Source: CAD feature listing. Evaluate the final solid. Frame: model axes, mm. A direction names the side the tool comes from. Round coordinates to 2 decimals unless told otherwise and drop trailing zeros. Loops run counter-clockwise (first coordinate to the right, second up) from the corner with the lowest first, then second, coordinate; pieces in that order, holes last. Notation, with made-up numbers: M 89,-39.75 L 136,-39.75 A12 cw 136,-30.75 Z; hole C 84,71 d4. An arc over 180 degrees is marked long. Answer as a JSON object with one key per item and string values.
from build123d import *

# Parameters (mm, degrees)
F1_DEPTH  = 15
F0_W      = 5
F0_H      = 13.750002
F2_DEPTH  = 12.5
F4_R      = 5
F5_R      = 5
F6_R      = 5
F7_R      = 3.275
F8_DEPTH  = 25
F3_W      = 2.5
F3_H      = 2
F9_DEPTH  = 50
F10_R     = 5
F11_DEPTH = 30


with BuildPart() as f1:
    # F0 (on Front) → F1 (new body, symmetric)
    with BuildSketch(Plane.XZ):
        Polygon((6.421984, -16.497303), (-11.078016, -16.497303), (-10.973849, -22.747303), (29.026151, -22.747303), (29.026151, -16.497303), (11.421984, -16.497303), align=None)
    extrude(amount=F1_DEPTH, both=True)

    # F0 (on Front) → F2 (join, symmetric)
    with BuildSketch(Plane.XZ):
        Polygon((6.421984, -16.497303), (-11.078016, -16.497303), (-10.973849, -22.747303), (29.026151, -22.747303), (29.026151, -16.497303), (11.421984, -16.497303), align=None)
        with Locations((8.921984, -9.622302)):
            Rectangle(F0_W, F0_H)
    extrude(amount=F2_DEPTH, both=True)

    # F4
    f4_edges = [f1.edges().sort_by_distance(p)[0] for p in [
        (29.026151, -15, -19.622303),
    ]]
    fillet(f4_edges, radius=F4_R)

    # F5
    f5_edges = [f1.edges().sort_by_distance(p)[0] for p in [
        (29.026151, 15, -19.622303),
        (-11.025932, -15, -19.622303),
        (-11.025932, 15, -19.622303),
    ]]
    fillet(f5_edges, radius=F5_R)

    # F6
    f6_edges = [f1.edges().sort_by_distance(p)[0] for p in [
        (8.921984, 12.5, -2.747301),
        (8.921984, -12.5, -2.747301),
    ]]
    fillet(f6_edges, radius=F6_R)

    # F7 (on Top) → F8 (cut)
    with BuildSketch(Plane.XY):
        with Locations((22.092594, 8.45)):
            Circle(F7_R)
        with Locations((21.753448, -8.45)):
            Circle(F7_R)
    extrude(amount=-F8_DEPTH, mode=Mode.SUBTRACT)

    # F3 (on Front) → F9 (cut, symmetric)
    with BuildSketch(Plane.XZ):
        with Locations((-0.973849, -21.747303)):
            Rectangle(F3_W, F3_H)
    extrude(amount=F9_DEPTH, both=True, mode=Mode.SUBTRACT)

    # F10 (on Right) → F11 (cut, symmetric)
    with BuildSketch(Plane.YZ):
        with Locations((0, -9.563591)):
            Circle(F10_R)
    extrude(amount=F11_DEPTH, both=True, mode=Mode.SUBTRACT)


solid = f1.part
Item 1: Contact query for flat-ended pins moving along their axis: pin 1 Ø11 at (y, z) = (-4, -10) entering from -X; pin 2 Ø8.5 at (x, y) = (21.75, -8.45) entering from +Z; pin 3 Ø0.6 at (y, z) = (7, -21.5) entering from -X; pin 4 Ø9 at (y, z) = (0, -9.56) entering from -X. Output: stop coordinate, or through.
Answer sheet:
{"pin 1": "stops at x = 6.42", "pin 2": "stops at z = -16.5", "pin 3": "stops at x = -11", "pin 4": "passes through"}
Item 2: Section D-D on x = -5.5. Return the cut outline in (y, z), then the cut area to 4 significant figures.
Answer sheet:
{"outline": "M -15,-22.75 L 15,-22.75 L 15,-16.5 L -15,-16.5 Z", "area": "187.5 mm²"}
Item 3: Pull-direction query (Y, two-part tool) for faces 4 (the cylindrical face through (8.957, -1.084, -14.445)), 5 (the cylindrical face through (-9.521, 13.574, -19.683)), 6 (the flat face through (-2.224, 0, -22)); classes: pulls with the +Y half, pulls with the -Y half, needs draft (parallel to the pull), parting line crosses it, or undercut.
Answer sheet:
{"face 4": "undercut", "face 5": "pulls with the +Y half", "face 6": "needs draft"}
Item 4: Section A-A on y = 0. Return the cut outline in (x, z), then the cut area to 3 significant figures.
Answer sheet:
{"outline": "M -11.08,-16.5 L -10.97,-22.75 L -2.22,-22.75 L -2.22,-20.75 L 0.28,-20.75 L 0.28,-22.75 L 29.03,-22.75 L 29.03,-16.5 L 11.42,-16.5 L 11.42,-14.56 L 6.42,-14.56 L 6.42,-16.5 Z; M 6.42,-4.56 L 11.42,-4.56 L 11.42,-2.75 L 6.42,-2.75 Z", "area": "264 mm²"}
Item 5: Section C-C on y = 4.5. Return the cut outline in (x, z), then the cut area to 3 significant figures.
Answer sheet:
{"outline": "M -11.08,-16.5 L -10.97,-22.75 L -2.22,-22.75 L -2.22,-20.75 L 0.28,-20.75 L 0.28,-22.75 L 29.03,-22.75 L 29.03,-16.5 L 11.42,-16.5 L 11.42,-11.74 L 6.42,-11.74 L 6.42,-16.5 Z; M 6.42,-7.38 L 11.42,-7.38 L 11.42,-2.75 L 6.42,-2.75 Z", "area": "292 mm²"}
Item 6: Section B-B on z = -6.5. Return the cut outline in (x, y).
Answer sheet:
{"outline": "M 6.42,-12.34 L 11.42,-12.34 L 11.42,-3.95 L 6.42,-3.95 Z; M 6.42,3.95 L 11.42,3.95 L 11.42,12.34 L 6.42,12.34 Z"}
Item 7: Access query for faces 1 (the cylindrical face through (-9.521, -13.574, -19.683)), 2 (the flat face through (6.422, -3, -14)), 3 (the flat face through (-1, 0, -20.747)). Directions: +Z, -Z, +X, -X, +Y, -Y. A direction counts if a zero-diameter tool reaches every point of the face in a straight line with its end or side. Return the directions, or none.
Answer sheet:
{"face 1": "-Z, -X, -Y", "face 2": "+Z, -X, +Y, -Y", "face 3": "-Z, +Y, -Y"}
Item 8: Line query: probe 1 along Y at (x, z) = (8.5, -9.5); probe 2 along X at (y, z) = (7, -19); probe 3 along X at (y, z) = (8.25, -12.25). Output: solid intervals per line, ascending. Write a range as from..to.
Answer sheet:
{"probe 1": "y = -12.5..-5, 5..12.5", "probe 2": "x = -11.04..19.16, 25.03..29.03", "probe 3": "x = 6.42..11.42"}
